```python
from build123d import *

# Parameters (mm, degrees)
BOSS_EXTRUDE1_DEPTH = 28
BOSS_EXTRUDE2_DEPTH = 5.5
CUT_EXTRUDE1_DEPTH  = 5.5
CUT_EXTRUDE2_DEPTH  = 8


with BuildPart() as part:
    # Sketch2 → Boss-Extrude1 (new body)
    with BuildSketch(Plane(origin=(0, 0, 0), x_dir=(1, 0, 0), z_dir=(0, 1, 0))):
        with BuildLine():
            Line((-248.771987083, 683.890458256), (-250.163612926, 673.36336753))
            Line((-250.163612926, 673.36336753), (-250.163612926, 669.53336753))
            Line((-250.163612926, 669.53336753), (-267.163612926, 669.53336753))
            Line((-267.163612926, 669.53336753), (-267.163612926, 664.78336753))
            Line((-267.163612926, 664.78336753), (-248.163612926, 664.78336753))
            Line((-248.163612926, 664.78336753), (-248.163612926, 626.928572815))
            Line((-248.163612926, 626.928572815), (-244.663612926, 626.928572815))
            Line((-244.663612926, 626.928572815), (-241.163612926, 626.928572815))
            Line((-241.163612926, 626.928572815), (-241.163612926, 664.990338865))
            Line((-241.163612926, 664.990338865), (-222.163612926, 664.990338865))
            Line((-222.163612926, 664.990338865), (-222.163612926, 669.53336753))
            Line((-222.163612926, 669.53336753), (-239.163612926, 669.53336753))
            Line((-239.163612926, 669.53336753), (-239.163612926, 673.362411263))
            Line((-239.163612926, 673.362411263), (-240.55523877, 683.890458256))
            ThreePointArc((-240.55523877, 683.890458256), (-244.663612926, 692.093561911), (-248.771987083, 683.890458256))
        make_face()
    extrude(amount=BOSS_EXTRUDE1_DEPTH)

    # Sketch6 → Boss-Extrude2 (add)
    with BuildSketch(Plane(origin=(0, 28, 0), x_dir=(1, 0, 0), z_dir=(0, 1, 0))):
        Polygon((-244.663612926, 673.362889397), (-242.163612926, 673.362889397), (-242.163612926, 657.990338865), (-244.663612926, 657.990338865), (-247.163612926, 657.990338865), (-247.163612926, 673.36310673), align=None)
    extrude(amount=BOSS_EXTRUDE2_DEPTH)

    # Sketch8 → Cut-Extrude1 (cut)
    with BuildSketch(Plane(origin=(0, 0, -669.53336753), x_dir=(-1, 0, 0), z_dir=(0, 0, -1))):
        Polygon((267.163612926, 20), (250.163612926, 25), (250.163612926, 28), (267.163612926, 28), align=None)
        Polygon((222.163612926, 20), (222.163612926, 28), (239.163612926, 28), (239.163612926, 25), align=None)
    extrude(amount=-CUT_EXTRUDE1_DEPTH, mode=Mode.SUBTRACT)

    # Sketch9 → Cut-Extrude2 (cut)
    with BuildSketch(Plane.ZY.offset(248.163612926)):
        Polygon((-626.928572815, 28), (-626.928572815, 23), (-656.928572815, 28), align=None)
    extrude(amount=-CUT_EXTRUDE2_DEPTH, mode=Mode.SUBTRACT)


solid = part.part
```
For this review, take the finished solid that the model builds, in its own axes (mm). A direction names the side the tool comes from. Coordinates: 2 decimals unless noted, no trailing zeros. Write each loop counter-clockwise with the first axis right and the second up, starting at its lowest first coordinate (ties: lowest second). Pieces come first, ordered by that corner, then holes.
(1) For pin 1 Ø14 at (y, z) = (13.5, -645.5) entering from +X; pin 2 Ø2 at (y, z) = (20.5, -656) entering from -X; pin 3 Ø2 at (y, z) = (6.5, -684.5) entering from -X; pin 4 Ø1.5 at (x, z) = (-258, -671) entering from -Y, all flat-tipped, find the tip position at first contact; note any pin that passes through.
(2) Tool access review of faces 5 (the face through (-250.164, 14, -671)), 6 (the face through (-259, 12, -669.533)), 7 (the face through (-247.164, 31, -666)): name each direction out of +Z, -Z, +X, -X, +Y, -Y from which nothing blocks a thin tool from reaching the whole face with its end or side.
(3) Add section C-C on x = -243. Give the boundary of the cut face in (y, z), then the cut area to 3 significant figures.
(4) The part is to be moulded in two halves that separate along Z. For faces 1 (the face through (-244.713, 25.465, -641.719)), 2 (the face through (-231, 12, -669.533)), 3 (the face through (-239.85, 13.8, -678.55)), 4 (the face through (-222.164, 10, -667)), say which applies: +Z half, -Z half, draft (parallel to the pull), parting line (faces both ways), or undercut.
(5) Add section B-B on z = -664. Give the boundary of the cut face in (x, y), then the cut area to 4 significant figures.
(6) Wall thickness on probe 1 along Z at (x, y) = (-238.5, 23); probe 2 along Y at (x, z) = (-240, -671); probe 3 along X at (y, z) = (4.5, -637): over which ranges is each line inside the solid? List them lowest first.
(7) Add section A-A on y = 11. Give the boundary of the cut face in (x, z).
(8) Add section D-D on y = 24. Give the boundary of the cut face in (x, z), then the cut area to 3 significant figures.
Answer sheet:
1. pin 1: stops at x = -241.16
1. pin 2: stops at x = -248.16
1. pin 3: stops at x = -249.58
1. pin 4: passes through
2. face 5: -Z, -X, +Y
2. face 6: -Z, -X, +Y, -Y
2. face 7: +Z, -Z, -X, +Y
3. outline: (0, -691.82) - (28, -691.82) - (28, -673.36) - (33.5, -673.36) - (33.5, -657.99) - (28, -657.99) - (28, -656.93) - (23, -626.93) - (0, -626.93) - close
3. area: 1,830 mm2
4. face 1: +Z half
4. face 2: -Z half
4. face 3: undercut
4. face 4: draft
5. outline: (-248.16, 0) - (-241.16, 0) - (-241.16, 28) - (-242.16, 28) - (-242.16, 33.5) - (-247.16, 33.5) - (-247.16, 28) - (-248.16, 28) - close
5. area: 223.5 mm2
6. probe 1: z = -669.53 to -664.99
6. probe 2: y = 0 to 28
6. probe 3: x = -248.16 to -241.16
7. outline: (-267.16, -669.53) - (-250.16, -669.53) - (-250.16, -673.36) - (-248.77, -683.89) arc R5.13 ccw (long way) to (-240.56, -683.89) - (-239.16, -673.36) - (-239.16, -669.53) - (-222.16, -669.53) - (-222.16, -664.99) - (-241.16, -664.99) - (-241.16, -626.93) - (-248.16, -626.93) - (-248.16, -664.78) - (-267.16, -664.78) - close
8. outline: (-253.56, -669.53) - (-250.16, -669.53) - (-250.16, -673.36) - (-248.77, -683.89) arc R5.13 ccw (long way) to (-240.56, -683.89) - (-239.16, -673.36) - (-239.16, -669.53) - (-235.76, -669.53) - (-235.76, -664.99) - (-241.16, -664.99) - (-241.16, -632.93) - (-248.16, -632.93) - (-248.16, -664.78) - (-253.56, -664.78) - close
8. area: 521 mm2
